Design review of the part built by this model. Coordinates are the model's own, in mm. Face numbers are marked on the shaded views. A direction names the side the tool comes from. Give positions to 0.01 mm unless a question says otherwise; leave off trailing zeros. Write each loop counter-clockwise with the first axis right and the second up, starting at its lowest first coordinate (ties: lowest second). Pieces come first, ordered by that corner, then holes. Notation, with made-up numbers: (-23, 40.25) -> (25, 40.25) arc R18 ccw to (25, 73.25) -> close; hole circle Ø11 at (13.25, 3). An arc over 180 degrees is marked (long way). Return JSON: item names as keys, results as strings. Group by question number.
from build123d import *

# Parameters (mm, degrees)
F1_DEPTH = 25.4
F3_R     = 15.7727010677
F5_R     = 8.5503070877
F6_DEPTH = 43.942


with BuildPart() as f1:
    # F0 (on Front) → F1 (new body, symmetric)
    with BuildSketch(Plane.XZ):
        with BuildLine():
            ThreePointArc((-25.4, 0), (0, 25.4), (25.4, 0))
            Line((25.4, 0), (25.4, -38.1))
            Line((25.4, -38.1), (44.45, -38.1))
            Line((44.45, -38.1), (44.45, 0))
            ThreePointArc((44.45, 0), (0, 44.45), (-44.45, 0))
            Line((-44.45, 0), (-44.45, -38.1))
            Line((-44.45, -38.1), (-25.4, -38.1))
            Line((-25.4, -38.1), (-25.4, 0))
        make_face()
    extrude(amount=F1_DEPTH, both=True)

    # F3 (on offset) → F4 (join, up to the next surface of F1)
    with BuildSketch(Plane.XY.offset(90.17)):
        Circle(F3_R)
    extrude(until=Until.NEXT, dir=(0, 0, -1))

    # F5 (on offset) → F6 (join, symmetric)
    with BuildSketch(Plane.XY.offset(90.17)):
        Circle(F5_R)
    extrude(amount=F6_DEPTH, both=True)


solid = f1.part
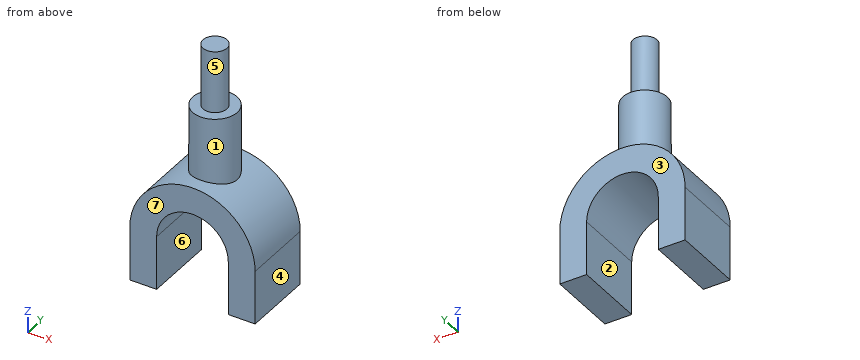
Q1. Take a section at C-C, the plane z = 18.5. Give the boundary of the cut face in (x, y), plus the area to 3 significant figures.
Q2. Take a section at D-D, the plane x = 5. Give the boundary of the cut face in (y, z), plus the area to 3 significant figures.
Q3. For L1, parallel to X at y = 5, z = -27; L2, parallel to Z at x = -36.5, y = 16.5; L3, parallel to X at y = 18.5, z = 21, list the stretches that pass through material, from the lowest coordinate up. Write a range as from..to.
Q4. Insertion check: pin 1 (4 mm diameter, centred on y = 0, z = 78, fed in from -X); pin 2 (3 mm diameter, centred on x = 5, z = 58.5, fed in from -Y); pin 3 (1 mm diameter, centred on x = 12, y = 17.5, fed in from +Z). Each pin has a flat end and moves straight along its axis. Give the tip position at first contact, or say it passes through.
Q5. Take a section at B-B, the plane y = 0. Give the boundary of the cut face in (x, z), plus the area to 3 significant figures.
Q6. Take a section at A-A, the plane z = -22. Give the boundary of the cut face in (x, y).
Q7. Tool access review of the marked faces 1, 2 and 3: name each direction out of +Z, -Z, +X, -X, +Y, -Y from which nothing blocks a thin tool from reaching the whole face with its end or side.
Q8. Mouldability with a two-part tool opening along X and no side actions: class the marked faces 4, 5, 6 and 7 as +X half, -X half, draft (parallel to the pull), parting line (faces both ways), or undercut.
Final values:
{
 "1": {"outline": "(-40.42, -25.4) -> (-17.4, -25.4) -> (-17.4, 25.4) -> (-40.42, 25.4) -> close; (17.4, -25.4) -> (40.42, -25.4) -> (40.42, 25.4) -> (17.4, 25.4) -> close", "area": "2,340 mm²"},
 "2": {"outline": "(-25.4, 24.9) -> (25.4, 24.9) -> (25.4, 44.17) -> (14.96, 44.17) -> (14.96, 90.17) -> (6.94, 90.17) -> (6.94, 134.11) -> (-6.94, 134.11) -> (-6.94, 90.17) -> (-14.96, 90.17) -> (-14.96, 44.17) -> (-25.4, 44.17) -> close", "area": "2,960 mm²"},
 "3": {"L1": "x = -44.45..-25.4, 25.4..44.45", "L2": "z = -38.1..25.37", "L3": "x = -39.18..-14.29, 14.29..39.18"},
 "4": {"pin 1": "stops at x = -15.77", "pin 2": "stops at y = -15.38", "pin 3": "stops at z = 42.94"},
 "5": {"outline": "(-44.45, -38.1) -> (-25.4, -38.1) -> (-25.4, 0) arc R25.4 cw to (25.4, 0) -> (25.4, -38.1) -> (44.45, -38.1) -> (44.45, 0) arc R44.45 ccw to (15.77, 41.56) -> (15.77, 90.17) -> (8.55, 90.17) -> (8.55, 134.11) -> (-8.55, 134.11) -> (-8.55, 90.17) -> (-15.77, 90.17) -> (-15.77, 41.56) arc R44.45 ccw to (-44.45, 0) -> close", "area": "5,770 mm²"},
 "6": {"outline": "(-44.45, -25.4) -> (-25.4, -25.4) -> (-25.4, 25.4) -> (-44.45, 25.4) -> close; (25.4, -25.4) -> (44.45, -25.4) -> (44.45, 25.4) -> (25.4, 25.4) -> close"},
 "7": {"face 1": "+Z", "face 2": "-Z, +Y, -Y", "face 3": "+Z, -Z, +X, -X, +Y"},
 "8": {"face 4": "+X half", "face 5": "parting line", "face 6": "undercut", "face 7": "draft"}
}
